Input: part model. Units: mm. Frame: model coordinates. Face numbers are marked on the shaded views. A direction names the side the tool comes from. Coordinates: 2 decimals unless noted, no trailing zeros. Write each loop counter-clockwise with the first axis right and the second up, starting at its lowest first coordinate (ties: lowest second). Pieces come first, ordered by that corner, then holes. Notation, with made-up numbers: M -15,49.25 L 22,49.25 A25 ccw 22,61.25 Z; hole C 19.25,-2.5 d5. An arc over 180 degrees is marked long. Use one line per item in the form item = value.
from build123d import *

# Parameters (mm, degrees)
ESQUISSE1_R             = 7.5
BOSS_EXTRU_1_DEPTH      = 10.5
BOSS_EXTRU_2_DEPTH      = 2
BOSS_EXTRU_2_DEPTH_BACK = 3.6
ESQUISSE2_R             = 10.1
ESQUISSE3_R             = 4.75
ENL_V_MAT_EXTRU_2_DEPTH = 6.999999999999999
ESQUISSE4_R             = 2.9
BOSS_EXTRU_3_DEPTH      = 6
CHANFREIN1_SIZE         = 3.75
CHANFREIN1_SIZE_2       = 7.5
ESQUISSE11_R            = 1.25
ENL_V_MAT_EXTRU_4_DEPTH = 7.5
ESQUISSE29_R            = 12
ESQUISSE29_R_2          = 10.1
BOSS_EXTRU_11_DEPTH     = 0.6
CONG_1_R                = 2


with BuildPart() as part:
    # Esquisse1 → Boss.-Extru.1 (new body)
    with BuildSketch(Plane(origin=(0, 0, 0), x_dir=(1, 0, 0), z_dir=(0, 1, 0))):
        with Locations(Location((0, 0, 0), (0, 0, 90))):
            Circle(ESQUISSE1_R)
    extrude(amount=BOSS_EXTRU_1_DEPTH)

    # Esquisse2 → Boss.-Extru.2 (add, two sides: drawn at the far end of the back side and taken through both)
    with BuildSketch(Plane.XZ.offset(-BOSS_EXTRU_2_DEPTH_BACK)):
        with Locations(Location((0, 0, 0), (0, 0, 270))):
            Circle(ESQUISSE2_R)
    extrude(amount=BOSS_EXTRU_2_DEPTH + BOSS_EXTRU_2_DEPTH_BACK)

    # Esquisse3 → Enlèv. mat.-Extru.2 (cut)
    with BuildSketch(Plane.XZ.offset(2)):
        with Locations(Location((0, 0, 0), (0, 0, 270))):
            Circle(ESQUISSE3_R)
    extrude(amount=-ENL_V_MAT_EXTRU_2_DEPTH, mode=Mode.SUBTRACT)

    # Esquisse4 → Boss.-Extru.3 (add)
    with BuildSketch(Plane.XZ.offset(-4.999999999999999)):
        with Locations(Location((0, 0, 0), (0, 0, 270))):
            Circle(ESQUISSE4_R)
    extrude(amount=BOSS_EXTRU_3_DEPTH)

    # Chanfrein1
    # the kernel refuses this chamfer: 7.5, 3.75 mm, written as the material it takes off along each edge
    with BuildSketch(Plane(origin=(0, -2, 0), x_dir=(-1.8e-16, 0, -1), z_dir=(-1, 0, 1.8e-16))) as chanfrein1_piece_1_section:
        Polygon((4.75 + CHANFREIN1_SIZE, 0), (4.75, -CHANFREIN1_SIZE_2), (4.75, 0), align=None)
    chanfrein1_piece_1 = revolve(axis=Axis((0, -2, 0), (0, -1, 0)), mode=Mode.PRIVATE)
    chanfrein1_piece_1 = split(chanfrein1_piece_1, bisect_by=Plane(origin=(2.06e-15, 4.999999999999999, 6.741862305399), z_dir=(0, -1, 0)), keep=Keep.TOP, mode=Mode.PRIVATE)
    add(chanfrein1_piece_1, mode=Mode.SUBTRACT)

    # Esquisse11 → Enlèv. mat.-Extru.4 (cut)
    with BuildSketch(Plane.XZ.offset(1.0000000000000009)):
        with Locations(Location((0, 0, 0), (0, 0, 270))):
            Circle(ESQUISSE11_R)
    extrude(amount=-ENL_V_MAT_EXTRU_4_DEPTH, mode=Mode.SUBTRACT)

    # Esquisse29 → Boss.-Extru.11 (add)
    with BuildSketch(Plane.XZ.offset(2)):
        with Locations(Location((0, 0, 0), (0, 0, 270))):
            Circle(ESQUISSE29_R)
        with Locations(Location((0, 0, 0), (0, 0, 270))):
            Circle(ESQUISSE29_R_2, mode=Mode.SUBTRACT)
    extrude(amount=-BOSS_EXTRU_11_DEPTH)

    # Congé1
    # the kernel refuses this fillet: 2 mm, written as the material it takes off along each edge
    with BuildSketch(Plane(origin=(0, -1.0000000000000009, 0), x_dir=(-1.8e-16, 0, -1), z_dir=(-1, 0, 1.8e-16))) as cong_1_piece_1:
        with BuildLine():
            CenterArc((3.25, -1.9691368667519222), CONG_1_R, 100.07865810778567, 79.92134189221433)
            Line((1.25, -1.9691368667519222), (1.21, -1.9691368667519222))
            Line((1.21, -1.9691368667519222), (1.21, 0))
            Line((1.21, 0), (1.25, 0.04000000000000004))
            ThreePointArc((1.25, 0.04000000000000004), (2.0750000000000344, 0.04000000000000004), (2.89300000000007, 0.03938273733464226))
            Line((2.89300000000007, 0.03938273733464226), (2.9000000000000687, -3.8836e-13))
        make_face()
    revolve(axis=Axis((0, -1.0000000000000009, 0), (0, -1, 0)), mode=Mode.SUBTRACT)


solid = part.part
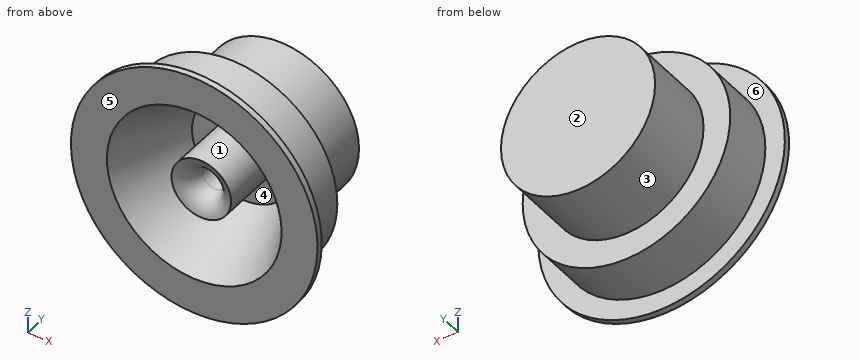
(1) Pull-direction query (Z, two-part tool) for the marked faces 1, 2 and 3; classes: pulls with the +Z half, pulls with the -Z half, needs draft (parallel to the pull), parting line crosses it, or undercut.
Computed:
face_1 = undercut
face_2 = needs draft
face_3 = parting line crosses it
(2) First-contact query: pin 1 Ø2 at (y, z) = (7, -1.5) entering from -X; pin 2 Ø1.5 at (x, y) = (-7, 0) entering from -Z; pin 3 Ø1.5 at (x, z) = (0, -2) entering from -Y. Flat tips, straight axial feed; report the tip coordinate or a pass-through.
Computed:
pin_1 = -7.48
pin_2 = -7.93
pin_3 = -0.97
(3) Line query: probe 1 along X at (y, z) = (4.2, 0); probe 2 along X at (y, z) = (2.5, 0); probe 3 along X at (y, z) = (2, -2). Output: solid intervals per line, ascending.
Computed:
probe_1 = -7.5 to -5.4, -2.9 to -1.25, 1.25 to 2.9, 5.4 to 7.5
probe_2 = -10.1 to -6.25, -2.9 to -1.25, 1.25 to 2.9, 6.25 to 10.1
probe_3 = -9.9 to -6.18, -2.1 to 2.1, 6.18 to 9.9
(4) Set-up query: the marked faces 4, 5 and 6. Return all of +Z, -Z, +X, -X, +Y, -Y with unobstructed straight access to the full face (end or side cutting, diameter ignored); none if empty.
Computed:
face_4 = -Y
face_5 = +Z, -Z, +X, -X, -Y
face_6 = +Y
(5) Section query C-C on y = 8.5. Return the cut outline in (x, z).
Computed:
outline = C 0,0 d15
(6) Section query A-A on x = 0. Return the cut outline in (y, z).
Computed:
outline = M -2,-12 L -1.4,-12 L -1.4,-10.1 L 3.6,-10.1 L 3.6,-7.5 L 10.5,-7.5 L 10.5,7.5 L 3.6,7.5 L 3.6,10.1 L -1.4,10.1 L -1.4,12 L -2,12 L -2,8.5 L 5,5 L 5,2.9 L -1,2.9 A2 ccw 0.97,1.25 L 6.5,1.25 L 6.5,-1.25 L 0.97,-1.25 A2 ccw -1,-2.9 L 5,-2.9 L 5,-5 L -2,-8.5 Z
(7) Section query D-D on x = -9.5. Return the cut outline in (y, z), plus the area to 3 significant figures.
Computed:
outline = M -2,-7.33 L -1.4,-7.33 L -1.4,-3.43 L 3.6,-3.43 L 3.6,3.43 L -1.4,3.43 L -1.4,7.33 L -2,7.33 Z
area = 43.1 mm^2
(8) Section query B-B on z = 0. Return the cut outline in (x, y).
Computed:
outline = M -12,-2 L -8.5,-2 L -5,5 L -2.9,5 L -2.9,-1 A2 ccw -1.25,0.97 L -1.25,6.5 L 1.25,6.5 L 1.25,0.97 A2 ccw 2.9,-1 L 2.9,5 L 5,5 L 8.5,-2 L 12,-2 L 12,-1.4 L 10.1,-1.4 L 10.1,3.6 L 7.5,3.6 L 7.5,10.5 L -7.5,10.5 L -7.5,3.6 L -10.1,3.6 L -10.1,-1.4 L -12,-1.4 Z
